Here's how the part is built. I have some questions about the finished solid (model axes, mm). Face numbers are marked on the shaded views. A direction names the side the tool comes from. Coordinates: 2 decimals unless noted, no trailing zeros. Write each loop counter-clockwise with the first axis right and the second up, starting at its lowest first coordinate (ties: lowest second). Pieces come first, ordered by that corner, then holes.
(1) Imagine slicing it at D-D, the plane y = 4.25. List the corners of the cut face in (x, z) for me, plus the area to 3 significant figures.
(2) Please list where these lines run through material, in increasing order: probe 1 along Y at (x, z) = (10, 5.5); probe 2 along X at (y, z) = (0.75, -8); probe 3 along Z at (x, y) = (0.5, -2.25).
(3) Imagine slicing it at C-C, the plane z = -1. List the corners of the cut face in (x, y) for me, plus the area to 3 significant figures.
(4) Imagine slicing it at B-B, the plane x = -12.5. List the corners of the cut face in (y, z) for me, plus the area to 3 significant figures.
(5) For pin 1 Ø3 at (x, y) = (10, -1) entering from +Z; pin 2 Ø12 at (x, z) = (1, -5) entering from -Y; pin 3 Ø5.5 at (x, y) = (-14.5, -2.5) entering from -Z; pin 4 Ø4 at (x, y) = (13, 0) entering from -Z, each with a flat end and sliding along its axis, tell me the tip position at first contact or that it passes through.
(6) Imagine slicing it at A-A, the plane y = -4.75. List the corners of the cut face in (x, z) for me.
(7) Which directions (+Z, -Z, +X, -X, +Y, -Y) give clear straight access to the entire face, cutting with the end or side of a thin tool? Please do the marked faces 1, 2 and 3.
```python
from build123d import *

# Parameters (mm, degrees)
CROQUIS1_W              = 11.8
CROQUIS1_H              = 32.4
SALIENTE_EXTRUIR1_DEPTH = 2.4
CROQUIS2_W              = 22.4
CROQUIS2_H              = 11.8
SALIENTE_EXTRUIR2_DEPTH = 4.5
CROQUIS3_R              = 5.905235569
SALIENTE_EXTRUIR3_DEPTH = 3.9
CROQUIS4_R              = 2.4
SALIENTE_EXTRUIR4_DEPTH = 3.3
CROQUIS5_W              = 22.4
CROQUIS5_H              = 11.8
SALIENTE_EXTRUIR5_DEPTH = 17


with BuildPart() as part:
    # Croquis1 → Saliente-Extruir1 (new body)
    with BuildSketch(Plane(origin=(0, 0, 0), x_dir=(0, 1, 0), z_dir=(0, 0, 1))):
        Rectangle(CROQUIS1_W, CROQUIS1_H)
    extrude(amount=SALIENTE_EXTRUIR1_DEPTH)

    # Croquis2 → Saliente-Extruir2 (add)
    with BuildSketch(Plane.XY.offset(2.4)):
        Rectangle(CROQUIS2_W, CROQUIS2_H)
    extrude(amount=SALIENTE_EXTRUIR2_DEPTH)

    # Croquis3 → Saliente-Extruir3 (add)
    with BuildSketch(Plane.XY.offset(6.9)):
        with Locations((5.294766752, -0.005235569)):
            Circle(CROQUIS3_R)
    extrude(amount=SALIENTE_EXTRUIR3_DEPTH)

    # Croquis4 → Saliente-Extruir4 (add)
    with BuildSketch(Plane.XY.offset(10.8)):
        with Locations((5.294766752, -0.005235569)):
            Circle(CROQUIS4_R)
    extrude(amount=SALIENTE_EXTRUIR4_DEPTH)

    # Croquis5 → Saliente-Extruir5 (add)
    with BuildSketch(Plane(origin=(0, 0, 0), x_dir=(1, 0, 0), z_dir=(0, 0, -1))):
        Rectangle(CROQUIS5_W, CROQUIS5_H)
    extrude(amount=SALIENTE_EXTRUIR5_DEPTH)


solid = part.part
```
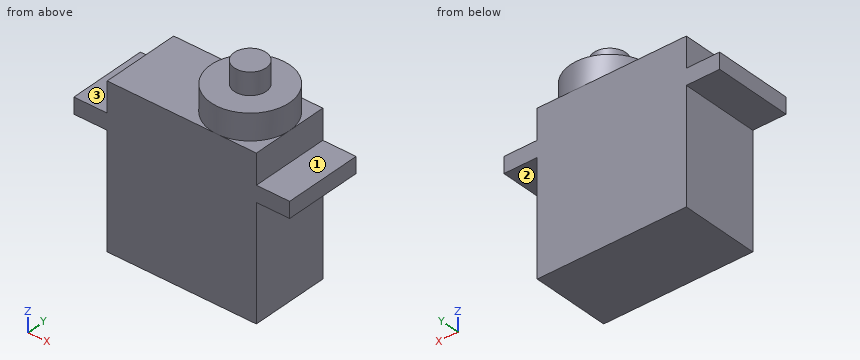
Recorded:
1. outline: (-16.2, 0) - (-11.2, 0) - (-11.2, -17) - (11.2, -17) - (11.2, 0) - (16.2, 0) - (16.2, 2.4) - (11.2, 2.4) - (11.2, 6.9) - (9.39, 6.9) - (9.39, 10.8) - (1.2, 10.8) - (1.2, 6.9) - (-11.2, 6.9) - (-11.2, 2.4) - (-16.2, 2.4) - close
1. area: 591 mm2
2. probe 1: y = -5.9 to 5.9
2. probe 2: x = -11.2 to 11.2
2. probe 3: z = -17 to 10.8
3. outline: (-11.2, -5.9) - (11.2, -5.9) - (11.2, 5.9) - (-11.2, 5.9) - close
3. area: 264 mm2
4. outline: (-5.9, 0) - (5.9, 0) - (5.9, 2.4) - (-5.9, 2.4) - close
4. area: 28.3 mm2
5. pin 1: stops at z = 10.8
5. pin 2: stops at y = -5.9
5. pin 3: stops at z = 0
5. pin 4: stops at z = -17
6. outline: (-16.2, 0) - (-11.2, 0) - (-11.2, -17) - (11.2, -17) - (11.2, 0) - (16.2, 0) - (16.2, 2.4) - (11.2, 2.4) - (11.2, 6.9) - (8.81, 6.9) - (8.81, 10.8) - (1.78, 10.8) - (1.78, 6.9) - (-11.2, 6.9) - (-11.2, 2.4) - (-16.2, 2.4) - close
7. face 1: +Z, +X, +Y, -Y
7. face 2: -Z, +X, +Y, -Y
7. face 3: +Z, -X, +Y, -Y
